from build123d import *

# Parameters (mm, degrees)
F0_R            = 10
F0_R_2          = 5.15
F1_DEPTH        = 2.8
F3_D            = 2.8
F3_COPIES_COUNT = 8
F4_SIZE         = 0.3


# Not quite as in the source:
# - a pattern or mirror of a feature is missing from the dataset's text; its kind, count and spacing are read off the source's solid


with BuildPart() as f1:
    # F0 (on Top) → F1 (new body)
    with BuildSketch(Plane.XY):
        Circle(F0_R)
        Circle(F0_R_2, mode=Mode.SUBTRACT)
    extrude(amount=F1_DEPTH)

    # F3 (through all)
    with Locations(Plane.XY.offset(2.8)):
        with Locations((0, 7)):
            f3 = Hole(F3_D / 2)

    # F3_copies: F3 ×8 about axis
    f3_copies_axis = Axis((0, 0, 0), (0, 0, 1))
    for i in range(1, F3_COPIES_COUNT):
        add(f3.rotate(f3_copies_axis, i * 360 / F3_COPIES_COUNT), mode=Mode.SUBTRACT)

    # F4
    f4_edges = [f1.edges().sort_by_distance(p)[0] for p in [
        (-5.15, 0, 0),
        (-10, 0, 0),
        (-5.15, 0, 2.8),
        (-10, 0, 2.8),
    ]]
    chamfer(f4_edges, length=F4_SIZE)


solid = f1.part
For this review, take the finished solid that the model builds, in its own axes (mm). Give positions to 0.01 mm unless a question says otherwise; leave off trailing zeros. Order: outer loops, then holes, each group sorted by start corner. A loop starts at its lowest first (then second) coordinate and runs counter-clockwise, first axis right, second up. Notation, with made-up numbers: (45, 48) - (53, 48) arc R17 cw to (53, 73) - close; hole circle Ø3 at (52, 1.5). An arc over 180 degrees is marked (long way). Answer as a JSON object with one key per item and string values. Group by question number.
Item 1: Take a section at A-A on x = 0. Give the boundary of the cut face in (y, z).
Item 2: Draft analysis for pull direction Y (two halves, no side actions). For faces 1 (the cylindrical face through (-2.17, -9.76, 1.38)), 2 (the cylindrical face through (-4.89, 6.35, 1.38)), 3 (the flat face through (6, -2, 2.8)), state which applies: pulls with the +Y half, pulls with the -Y half, needs draft (parallel to the pull), parting line crosses it, or undercut.
Item 3: Wall thickness on line 1 along X through (y, z) = (-4, 0.9); line 2 along Y through (x, z) = (6, 1.3); line 3 along Y through (x, z) = (4.25, 1.2): over which ranges is each line inside the solid? List them lowest first.
Item 4: Take a section at C-C on z = 0.7. Give the number of separate pieces and of enclosed holes in the cut face, and give its area (3 significant figures).
Item 5: Clearance check with a flat-ended pin moving along its axis: pin 1 Ø2 at (x, y) = (0, -7) entering from +Z. State where the tip first meets the part, or that it passes through.
Reported:
{
 "1": {"outline": "(-10, 0.3) - (-9.7, 0) - (-8.4, 0) - (-8.4, 2.8) - (-9.7, 2.8) - (-10, 2.5) - close; (-5.6, 0) - (-5.45, 0) - (-5.15, 0.3) - (-5.15, 2.5) - (-5.45, 2.8) - (-5.6, 2.8) - close; (5.15, 0.3) - (5.45, 0) - (5.6, 0) - (5.6, 2.8) - (5.45, 2.8) - (5.15, 2.5) - close; (8.4, 0) - (9.7, 0) - (10, 0.3) - (10, 2.5) - (9.7, 2.8) - (8.4, 2.8) - close"},
 "2": {"face 1": "parting line crosses it", "face 2": "undercut", "face 3": "needs draft"},
 "3": {"line 1": "-9.17 to -5.98, -3.92 to -3.24, 3.24 to 3.92, 5.98 to 9.17", "line 2": "-8 to -5.88, -4.02 to -0.98, 0.98 to 4.02, 5.88 to 8", "line 3": "-9.05 to -6.16, -3.74 to -2.91, 2.91 to 3.74, 6.16 to 9.05"},
 "4": {"separate pieces": "1", "enclosed holes": "9", "area": "182 mm^2"},
 "5": {"pin 1": "through"}
}
